Input: part model. Units: mm. Frame: model coordinates. A direction names the side the tool comes from. Coordinates: 2 decimals unless noted, no trailing zeros. Write each loop counter-clockwise with the first axis right and the second up, starting at its lowest first coordinate (ties: lowest second). Pieces come first, ordered by that corner, then holes.
1) Line query: L1, parallel to Z at x = 36, y = 6; L2, parallel to X at y = 5.75, z = 120; L3, parallel to X at y = 0.75, z = -99.5. Output: solid intervals per line, ascending.
2) Section query C-C (x = 36). Output: boundary loops of the cut face in (y, z).
3) Set-up query: faces 1 (the flat face through (78, 4, -57.5)), 2 (the flat face through (7, 0, 3)), 3 (the flat face through (77, 4, 57.5)). Return all of +Z, -Z, +X, -X, +Y, -Y with unobstructed straight access to the full face (end or side cutting, diameter ignored); none if empty.
4) Section query A-A (z = -120). Output: boundary loops of the cut face in (x, y).
5) Section query B-B (y = 5.75). Output: boundary loops of the cut face in (x, z).
6) Draft query along X for faces 4 (the flat face through (1, 4, 200)), 5 (the cylindrical face through (39.83, 4.056, 170.763)), 6 (the flat face through (-56, 4, 3)). Return one class per face: pulls with the +X half, pulls with the -X half, needs draft (parallel to the pull), parting line crosses it, or undercut.
7) Pin query (flat end, axial travel): pin 1 Ø2 at (y, z) = (4.5, -138.5) entering from +X. Return the tip coordinate at first contact, or that it passes through.
8) Section query D-D (z = -71.5). Output: boundary loops of the cut face in (x, y), then the cut area to 3 significant figures.
Autodesk Inventor part; units mm, degrees
ref_plane "YZ Plane" through (0, 0, 0) normal (1, 0, 0) x (0, 1, 0)
ref_plane "XZ Plane" through (0, 0, 0) normal (0, 1, 0) x (-1, 0, 0)
ref_plane "XY Plane" through (0, 0, 0) normal (0, 0, 1) x (1, 0, 0)
sketch "Sketch1" plane through (0, 0, 0) normal (0, 1, 0) x (-1, 0, 0)
  line L0 (56, -200) -> (-56, -200)
  line L1 (-56, -200) -> (-56, 200)
  line L2 (-56, 200) -> (56, 200)
  line L3 (56, 200) -> (56, -200)
  line L4 (56, -200) -> (-56, 200) construction
  line L5 (-56, -200) -> (56, 200) construction
  line L6 (-56, 57.5) -> (-103, 57.5)
  line L7 (-103, 57.5) -> (-103, -57.5)
  line L8 (-103, -57.5) -> (-56, -57.5)
  point P0 (0, 0)
  point P1 (0, 0)
  point P2 (-103, 0)
  point P3 (-56, 0)
  dimension "d16" = 112
  dimension "d17" = 400
  dimension "d24" = 47
  dimension "d25" = 115
extrude "Plate1" add sketch "Sketch1" along normal blind 8
sketch "Sketch2" plane through (0, 0, 0) normal (0, -1, 0) x (1, 0, 0)
  line L0 (36, 180) -> (36, -180) construction
  line L1 (-56, -200) -> (56, -200)
  line L2 (56, -200) -> (56, -57.5)
  line L3 (56, 200) -> (-56, 200)
  line L4 (-56, 200) -> (-56, -200)
  line L5 (103, -57.5) -> (56, -57.5)
  line L6 (103, 57.5) -> (103, -57.5)
  line L7 (56, 57.5) -> (103, 57.5)
  line L8 (56, 57.5) -> (56, 200)
  point P0 (36, 0)
  point P1 (36, 0)
  point P2 (0, 0)
  point P3 (36, 120)
  point P4 (36, -120)
  dimension "d19" = 20
  dimension "d20" = 20
  dimension "d21" = 360
  dimension "d22" = 120
  dimension "d23" = 120
hole "Hole1" at (36, 0, 180) at (36, 0, -180) at (36, 0, -120) at (36, 0, 120) direction (0, 1, 0) diameter 20 end through all
fillet "Fillet1" radius 4 2 edges at (103, 4, 57.5) (103, 4, -57.5)
equation "\"d20\" = d19"
equation "\"d3\" = d19"
equation "\"d8\" = Thickness"
equation "\"d2\" = Thickness"
equation "\"BendRadius\" = Thickness"
equation "\"BendReliefWidth\" = Thickness"
equation "\"BendReliefDepth\" = 0.5 * Thickness"
equation "\"CornerReliefSize\" = 4 * Thickness"
equation "\"MinimumRemnant\" = 2 * Thickness"
equation "\"TransitionRadius\" = BendRadius"
equation "\"JacobiRadiusSize\" = BendRadius"
equation "\"GapSize\" = Thickness"
properties part number "Ухо на швеллер пямое_CPY"
Answer:
1. L1: z = -200 to -190, -170 to -130, -110 to 110, 130 to 170, 190 to 200
1. L2: x = -56 to 26, 46 to 56
1. L3: x = -56 to 56
2. outline: (0, -200) - (8, -200) - (8, -190) - (0, -190) - close; (0, -170) - (8, -170) - (8, -130) - (0, -130) - close; (0, -110) - (8, -110) - (8, 110) - (0, 110) - close; (0, 130) - (8, 130) - (8, 170) - (0, 170) - close; (0, 190) - (8, 190) - (8, 200) - (0, 200) - close
3. face 1: -Z, +X, +Y, -Y
3. face 2: +Z, -Z, +X, -X, -Y
3. face 3: +Z, +X, +Y, -Y
4. outline: (-56, 0) - (26, 0) - (26, 8) - (-56, 8) - close; (46, 0) - (56, 0) - (56, 8) - (46, 8) - close
5. outline: (-56, -200) - (56, -200) - (56, -57.5) - (99, -57.5) arc R4 ccw to (103, -53.5) - (103, 53.5) arc R4 ccw to (99, 57.5) - (56, 57.5) - (56, 200) - (-56, 200) - close; hole circle Ø20 at (36, -180); hole circle Ø20 at (36, -120); hole circle Ø20 at (36, 120); hole circle Ø20 at (36, 180)
6. face 4: needs draft
6. face 5: undercut
6. face 6: pulls with the -X half
7. pin 1: stops at x = 56
8. outline: (-56, 0) - (56, 0) - (56, 8) - (-56, 8) - close
8. area: 896 mm2
